from build123d import *

# Parameters (mm, degrees)
SKETCH1_W                                        = 74.6252
SKETCH1_H                                        = 63.5
BOSS_EXTRUDE1_DEPTH                              = 14.224
CBORE_FOR_1_4_SOCKET_HEAD_CAP_SCREW1_D           = 8.0264
CBORE_FOR_1_4_SOCKET_HEAD_CAP_SCREW1_CBORE_D     = 11.0998
CBORE_FOR_1_4_SOCKET_HEAD_CAP_SCREW1_CBORE_DEPTH = 7.874
SKETCH9_W                                        = 25.4
SKETCH9_H                                        = 63.5
CUT_EXTRUDE1_DEPTH                               = 1.524
SKETCH10_R                                       = 11.1125
CUT_EXTRUDE2_DEPTH                               = 1.397


with BuildPart() as part:
    # Sketch1 → Boss-Extrude1 (new body)
    with BuildSketch(Plane.XY):
        with Locations((37.3126, 31.75)):
            Rectangle(SKETCH1_W, SKETCH1_H)
    extrude(amount=BOSS_EXTRUDE1_DEPTH)

    # CBORE for 1/4 Socket Head Cap Screw1 (through all)
    with Locations(Plane.XY.offset(14.224)):
        with Locations((37.3126, 31.75)):
            CounterBoreHole(CBORE_FOR_1_4_SOCKET_HEAD_CAP_SCREW1_D / 2, CBORE_FOR_1_4_SOCKET_HEAD_CAP_SCREW1_CBORE_D / 2, CBORE_FOR_1_4_SOCKET_HEAD_CAP_SCREW1_CBORE_DEPTH)

    # Sketch9 → Cut-Extrude1 (cut)
    with BuildSketch(Plane.XY.offset(14.224)):
        with Locations((37.3126, 31.75)):
            Rectangle(SKETCH9_W, SKETCH9_H)
    extrude(amount=-CUT_EXTRUDE1_DEPTH, mode=Mode.SUBTRACT)

    # Sketch10 → Cut-Extrude2 (cut)
    with BuildSketch(Plane(origin=(0, 0, 0), x_dir=(-1, 0, 0), z_dir=(0, 0, -1))):
        with Locations((-37.3126, 31.75)):
            Circle(SKETCH10_R)
    extrude(amount=-CUT_EXTRUDE2_DEPTH, mode=Mode.SUBTRACT)


solid = part.part
Model file for the job. Use its own axes, mm. A direction names the side the tool comes from. Give positions to 0.01 mm unless a question says otherwise; leave off trailing zeros. Write each loop counter-clockwise with the first axis right and the second up, starting at its lowest first coordinate (ties: lowest second). Pieces come first, ordered by that corner, then holes. Notation, with made-up numbers: M 44.25,35.25 L 49.25,35.25 A16 cw 49.25,52.25 Z; hole C -31,56.25 d1. An arc over 180 degrees is marked long. One line per item, written item: value. Start each with the question number.
Q1. 3-axis set-ups, long thin cutter, end or side, ignore diameter. For faces 5 (the flat face through (37, 0, 7)), 6 (the cylindrical face through (33.22, 35.5, 9.57)), 7 (the flat face through (33, 32, 1.397)), 8 (the flat face through (24.613, 31, 13)): which of +Z, -Z, +X, -X, +Y, -Y reach the whole face in a straight line?
Q2. Probe probe 1 along X at (y, z) = (7, 13.25); probe 2 along Z at (x, y) = (25, 45); probe 3 along X at (y, z) = (28.5, 7.5). List the from-to ranges inside material, lowest first. Write a range as [from, to].
Q3. Saw through at A-A, the plane y = 31.75. Write the cut outline in (x, z), plus the area to 3 significant figures.
Q4. Drop flat-ended pins along their axis: pin 1 Ø9 at (x, y) = (37.31, 31.75) entering from -Z; pin 2 Ø3.5 at (x, y) = (36.5, 34) entering from +Z; pin 3 Ø12.5 at (x, y) = (32, 32.5) entering from +Z. Give the stop position or say it passes through.
Q5. Saw through at B-B, the plane z = 8.25. Write the cut outline in (x, y), plus the area to 3 significant figures.
Q6. Two-plate mould, pull along X, no slides. Class faces 1 (the flat face through (28, 39, 0)), 2 (the cylindrical face through (48.414, 32.239, 0.689)), 3 (the flat face through (74.625, 31, 7)), 4 (the flat face through (0, 31, 7)): +X half, -X half, draft (parallel to the pull), parting line (faces both ways), or undercut.
Q7. Saw through at C-C, the plane y = 46. Write the cut outline in (x, z).
Output values:
1. face 5: +Z, -Z, +X, -X, -Y
1. face 6: +Z
1. face 7: -Z
1. face 8: +Z, +Y, -Y
2. probe 1: x = [0, 24.61], [50.01, 74.63]
2. probe 2: z = [0, 12.7]
2. probe 3: x = [0, 32.81], [41.81, 74.63]
3. outline: M 0,0 L 26.2,0 L 26.2,1.4 L 33.3,1.4 L 33.3,6.35 L 31.76,6.35 L 31.76,12.7 L 24.61,12.7 L 24.61,14.22 L 0,14.22 Z; M 41.33,1.4 L 48.43,1.4 L 48.43,0 L 74.63,0 L 74.63,14.22 L 50.01,14.22 L 50.01,12.7 L 42.86,12.7 L 42.86,6.35 L 41.33,6.35 Z
3. area: 881 mm²
4. pin 1: stops at z = 1.4
4. pin 2: stops at z = 6.35
4. pin 3: stops at z = 12.7
5. outline: M 0,0 L 74.63,0 L 74.63,63.5 L 0,63.5 Z; hole C 37.31,31.75 d11.1
5. area: 4,640 mm²
6. face 1: draft
6. face 2: undercut
6. face 3: +X half
6. face 4: -X half
7. outline: M 0,0 L 74.63,0 L 74.63,14.22 L 50.01,14.22 L 50.01,12.7 L 24.61,12.7 L 24.61,14.22 L 0,14.22 Z
